from build123d import *

# Parameters (mm, degrees)
SKETCH_1_W      = 60
SKETCH_1_H      = 100
SKETCH_1_R      = 2.5
SKETCH_1_R_2    = 2
SKETCH_1_R_3    = 3.5
EXTRUDE_1_DEPTH = 3


with BuildPart() as part:
    # Эскиз1 → Бобышка-Вытянуть1 (new body)
    with BuildSketch(Plane.XY):
        with Locations((-30, 50)):
            Rectangle(SKETCH_1_W, SKETCH_1_H)
        with Locations((-30, 50)):
            Circle(SKETCH_1_R, mode=Mode.SUBTRACT)
        with Locations((-21, 50)):
            Circle(SKETCH_1_R, mode=Mode.SUBTRACT)
        with Locations(Location((-39, 50, 0), (0, 0, 180))):
            Circle(SKETCH_1_R, mode=Mode.SUBTRACT)
        with Locations((-30, 41)):
            Circle(SKETCH_1_R, mode=Mode.SUBTRACT)
        with Locations(Location((-30, 59, 0), (0, 0, 180))):
            Circle(SKETCH_1_R, mode=Mode.SUBTRACT)
        with Locations((-50, 93)):
            Circle(SKETCH_1_R_2, mode=Mode.SUBTRACT)
        with Locations((-50, 83)):
            Circle(SKETCH_1_R_2, mode=Mode.SUBTRACT)
        with Locations(Location((-10, 83, 0), (0, 0, 180))):
            Circle(SKETCH_1_R_2, mode=Mode.SUBTRACT)
        with Locations(Location((-10, 93, 0), (0, 0, 180))):
            Circle(SKETCH_1_R_2, mode=Mode.SUBTRACT)
        with Locations((-10, 17)):
            Circle(SKETCH_1_R_2, mode=Mode.SUBTRACT)
        with Locations((-10, 7)):
            Circle(SKETCH_1_R_2, mode=Mode.SUBTRACT)
        with Locations(Location((-50, 7, 0), (0, 0, 180))):
            Circle(SKETCH_1_R_2, mode=Mode.SUBTRACT)
        with Locations(Location((-50, 17, 0), (0, 0, 180))):
            Circle(SKETCH_1_R_2, mode=Mode.SUBTRACT)
        with Locations((-48, 50)):
            Circle(SKETCH_1_R, mode=Mode.SUBTRACT)
        with Locations((-12, 50)):
            Circle(SKETCH_1_R_3, mode=Mode.SUBTRACT)
    extrude(amount=EXTRUDE_1_DEPTH)


solid = part.part
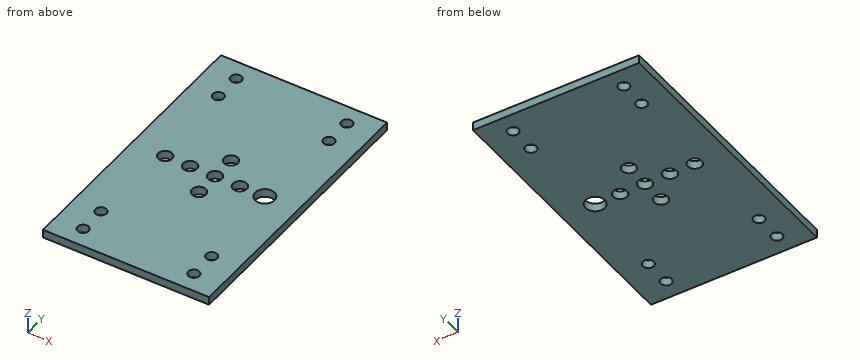
Verification items for the finished model (mm, model axes). Coordinates: 2 decimals unless noted, no trailing zeros. Order: outer loops, then holes, each group sorted by start corner. A loop starts at its lowest first (then second) coordinate and runs counter-clockwise, first axis right, second up.
1. Scan lines: line 1 (Y direction, x = -30, z = 2.4); line 2 (Y direction, x = -10, z = 2.4); line 3 (Y direction, x = -29.5, z = 2.7). Record each from-to range of solid material in increasing order.
Results found:
line 1: y = 0 to 38.5, 43.5 to 47.5, 52.5 to 56.5, 61.5 to 100
line 2: y = 0 to 5, 9 to 15, 19 to 47.13, 52.87 to 81, 85 to 91, 95 to 100
line 3: y = 0 to 38.55, 43.45 to 47.55, 52.45 to 56.55, 61.45 to 100
2. Sectioned sample at B-B, the plane y = 17. Record the cut outline in (x, z).
Results found:
outline: (-60, 0) - (-52, 0) - (-52, 3) - (-60, 3) - close; (-48, 0) - (-12, 0) - (-12, 3) - (-48, 3) - close; (-8, 0) - (0, 0) - (0, 3) - (-8, 3) - close
3. Sectioned sample at C-C, the plane y = 41. Record the cut outline in (x, z).
Results found:
outline: (-60, 0) - (-32.5, 0) - (-32.5, 3) - (-60, 3) - close; (-27.5, 0) - (0, 0) - (0, 3) - (-27.5, 3) - close
4. Sectioned sample at A-A, the plane z = 1.2. Give the number of separate pieces and of enclosed holes in the cut face, and give its area (3 significant figures).
Results found:
separate pieces: 1
enclosed holes: 15
area: 5,740 mm2
